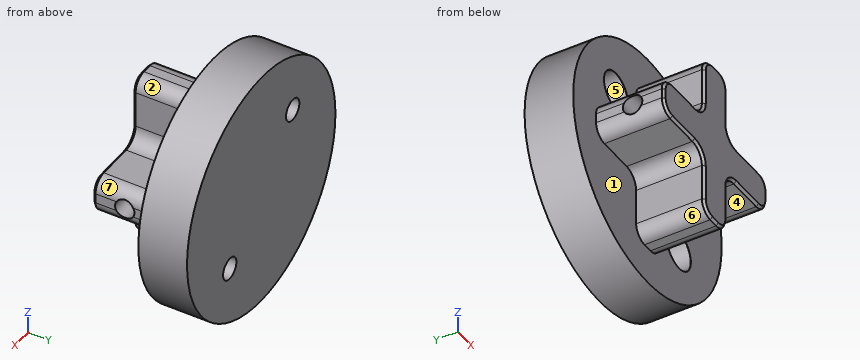
from build123d import *

# Parameters (mm, degrees)
SKETCH1_R                                    = 25
BOSS_EXTRUDE1_DEPTH                          = 25
BOSS_EXTRUDE2_DEPTH                          = 14
SKETCH3_R                                    = 2
CUT_EXTRUDE1_DEPTH                           = 56.129756031
CHAMFER1_SIZE                                = 0.5
CUT_EXTRUDE3_DEPTH                           = 15
CBORE_FOR_M4_HEX_SOCKET_HEAD_CAP_SCR_2_COUNT = 2
CBORE_FOR_M4_HEX_SOCKET_HEAD_CAP_SCR_2_PITCH = 30
CUT_EXTRUDE4_START                           = -15
CUT_EXTRUDE4_DEPTH                           = 15


with BuildPart() as part:
    # Sketch1 → Boss-Extrude1 (new body)
    with BuildSketch(Plane(origin=(0, 0, 0), x_dir=(1, 0, 0), z_dir=(0, 1, 0))):
        with Locations(Location((0, 0, 0), (0, 0, 270))):
            Circle(SKETCH1_R)
    extrude(amount=BOSS_EXTRUDE1_DEPTH)

    # Sketch2 → Boss-Extrude2 (add)
    with BuildSketch(Plane.XZ):
        with BuildLine():
            Line((-17.3, 1), (-17.3, -1))
            ThreePointArc((-17.3, -1), (-16.479898987, -2.979898987), (-14.5, -3.8))
            Line((-14.5, -3.8), (-7, -3.8))
            ThreePointArc((-7, -3.8), (-4.7372583, -4.7372583), (-3.8, -7))
            Line((-3.8, -7), (-3.8, -14.5))
            ThreePointArc((-3.8, -14.5), (-2.979898987, -16.479898987), (-1, -17.3))
            Line((-1, -17.3), (1, -17.3))
            ThreePointArc((1, -17.3), (2.979898987, -16.479898987), (3.8, -14.5))
            Line((3.8, -14.5), (3.8, -7))
            ThreePointArc((3.8, -7), (4.7372583, -4.7372583), (7, -3.8))
            Line((7, -3.8), (14.5, -3.8))
            ThreePointArc((14.5, -3.8), (16.479898987, -2.979898987), (17.3, -1))
            Line((17.3, -1), (17.3, 1))
            ThreePointArc((17.3, 1), (16.479898987, 2.979898987), (14.5, 3.8))
            Line((14.5, 3.8), (7, 3.8))
            ThreePointArc((7, 3.8), (4.7372583, 4.7372583), (3.8, 7))
            Line((3.8, 7), (3.8, 14.5))
            ThreePointArc((3.8, 14.5), (2.979898987, 16.479898987), (1, 17.3))
            Line((1, 17.3), (-1, 17.3))
            ThreePointArc((-1, 17.3), (-2.979898987, 16.479898987), (-3.8, 14.5))
            Line((-3.8, 14.5), (-3.8, 7))
            ThreePointArc((-3.8, 7), (-4.7372583, 4.7372583), (-7, 3.8))
            Line((-7, 3.8), (-14.5, 3.8))
            ThreePointArc((-14.5, 3.8), (-16.479898987, 2.979898987), (-17.3, 1))
        make_face()
    extrude(amount=BOSS_EXTRUDE2_DEPTH)

    # Sketch3 → Cut-Extrude1 (cut, through all)
    with BuildSketch(Plane.ZY.offset(17.3)):
        with Locations(Location((0, -7.5, 0), (0, 0, 60))):
            Circle(SKETCH3_R)
    extrude(amount=-CUT_EXTRUDE1_DEPTH, mode=Mode.SUBTRACT)

    # Chamfer1
    chamfer1_edges = [part.edges().sort_by_distance(p)[0] for p in [
        (-16.479898987, -14, -2.979898987),
        (-10.75, -14, -3.8),
        (-4.7372583, -14, -4.7372583),
        (-3.8, -14, -10.75),
        (-2.979898987, -14, -16.479898987),
        (0, -14, -17.3),
        (2.979898987, -14, -16.479898987),
        (3.8, -14, -10.75),
        (4.7372583, -14, -4.7372583),
        (10.75, -14, -3.8),
        (16.479898987, -14, -2.979898987),
        (17.3, -14, 0),
        (16.479898987, -14, 2.979898987),
        (10.75, -14, 3.8),
        (4.7372583, -14, 4.7372583),
        (3.8, -14, 10.75),
        (2.979898987, -14, 16.479898987),
        (0, -14, 17.3),
        (-2.979898987, -14, 16.479898987),
        (-3.8, -14, 10.75),
        (-4.7372583, -14, 4.7372583),
        (-10.75, -14, 3.8),
        (-16.479898987, -14, 2.979898987),
        (-17.3, -14, 0),
    ]]
    chamfer(chamfer1_edges, length=CHAMFER1_SIZE)

    # Sketch7 → Cut-Extrude3 (cut)
    with BuildSketch(Plane(origin=(0, 25, 0), x_dir=(1, 0, 0), z_dir=(0, 1, 0))):
        with BuildLine():
            Line((-25.358862505, -19.065612153), (19.065612153, 25.358862505))
            ThreePointArc((19.065612153, 25.358862505), (25.358862505, 25.358862505), (25.358862505, 19.065612153))
            Line((25.358862505, 19.065612153), (-19.065612153, -25.358862505))
            ThreePointArc((-19.065612153, -25.358862505), (-25.358862505, -25.358862505), (-25.358862505, -19.065612153))
        make_face()
    extrude(amount=-CUT_EXTRUDE3_DEPTH, mode=Mode.SUBTRACT)

    # Sketch6 → CBORE for M4 Hex Socket Head Cap Screw1 (revolve, cut)
    with BuildSketch(Plane(origin=(10.606601718, 0, -10.606601718), x_dir=(0, 0, -1), z_dir=(1, 0, 0))):
        Polygon((0, 0), (0, 14.351936393), (2.25, 13), (2.25, 4.4), (4, 4.4), (4, 0.025), (4.025, 0), align=None)
    cbore_for_m4_hex_socket_head_cap_screw1 = revolve(axis=Axis((10.606601718, -6.35, -10.606601718), (0, 1, 0)), mode=Mode.SUBTRACT)

    # CBORE for M4 Hex Socket Head Cap Scr 2: CBORE for M4 Hex Socket Head Cap Screw1 ×2
    with Locations(*[Vector(-0.707106781186549, 0, 0.7071067811865461) * (i * CBORE_FOR_M4_HEX_SOCKET_HEAD_CAP_SCR_2_PITCH) for i in range(1, CBORE_FOR_M4_HEX_SOCKET_HEAD_CAP_SCR_2_COUNT)]):
        add(cbore_for_m4_hex_socket_head_cap_screw1, mode=Mode.SUBTRACT)

    # Sketch8 → Cut-Extrude4 (cut)
    with BuildSketch(Plane(origin=(0, 25, 0), x_dir=(1, 0, 0), z_dir=(0, 1, 0)).offset(CUT_EXTRUDE4_START)):
        with BuildLine():
            Line((20.541990938, 14.248740586), (-14.248740586, -20.541990938))
            ThreePointArc((-14.248740586, -20.541990938), (17.67766953, -17.67766953), (20.541990938, 14.248740586))
        make_face()
        with BuildLine():
            Line((-20.541990938, -14.248740586), (14.248740586, 20.541990938))
            ThreePointArc((14.248740586, 20.541990938), (-17.67766953, 17.67766953), (-20.541990938, -14.248740586))
        make_face()
    extrude(amount=CUT_EXTRUDE4_DEPTH, mode=Mode.SUBTRACT)


solid = part.part
Geometry: final body of the model. Coordinates: model frame, mm. Face numbers are marked on the shaded views. A direction names the side the tool comes from. Give positions to 0.01 mm unless a question says otherwise; leave off trailing zeros. Write each loop counter-clockwise with the first axis right and the second up, starting at its lowest first coordinate (ties: lowest second). Pieces come first, ordered by that corner, then holes. Notation, with made-up numbers: M 24.25,64 L 70.25,64 A14 ccw 70.25,69 Z; hole C 45,7.5 d7. An arc over 180 degrees is marked long. Answer in a Markdown table with one row per item. Add a question column.
(1) Section A-A on x = 0. Return loops of the section in (y, z).
(2) Mould query, pull axis Z, two halves, no side actions, for the marked faces 5, 6 and 7. Classes: +Z half, -Z half, draft (parallel to the pull), parting line (faces both ways), or undercut.
(3) Section D-D on y = -7.5. Return loops of the section in (x, z), and give its area (3 significant figures).
(4) First-contact query: pin 1 (2 mm diameter, centred on x = -10, z = 8, fed in from -Y); pin 2 (8 mm diameter, centred on x = -11.5, y = -5.5, fed in from -Z); pin 3 (2 mm diameter, centred on y = -5, z = -14.5, fed in from -X); pin 4 (2.5 mm diameter, centred on y = -7.5, z = 0, fed in from -X). Flat tips, straight axial feed; report the tip coordinate or a pass-through.
(5) Section C-C on y = -11.5. Return loops of the section in (x, z).
(6) Section B-B on z = 0. Return loops of the section in (x, y).
(7) Reachability of the marked faces 1, 2, 3 and 4 from +Z, -Z, +X, -X, +Y, -Y: full face, straight path, thin tool, end or side. Return the list, or none.
(8) Ray query, line 1 (Y direction, x = 9, z = 0); line 2 (Y direction, x = -17.5, z = -2); line 3 (Z direction, x = -14, y = -1.75). Return the intervals inside material, ascending.
Result set:
| question | item | result |
|---|---|---|
| 1 | outline | M -14,-16.8 L -13.5,-17.3 L 0,-17.3 L 0,-25 L 10,-25 L 10,25 L 0,25 L 0,17.3 L -13.5,17.3 L -14,16.8 Z; hole C -7.5,0 d4 |
| 2 | face 5 | undercut |
| 2 | face 6 | -Z half |
| 2 | face 7 | +Z half |
| 3 | outline | M -17.12,-2 A2.8 ccw -14.5,-3.8 L -7,-3.8 A3.2 cw -3.8,-7 L -3.8,-14.5 A2.8 ccw -1,-17.3 L 1,-17.3 A2.8 ccw 3.8,-14.5 L 3.8,-7 A3.2 cw 7,-3.8 L 14.5,-3.8 A2.8 ccw 17.12,-2 Z; M -17.12,2 L 17.12,2 A2.8 ccw 14.5,3.8 L 7,3.8 A3.2 cw 3.8,7 L 3.8,14.5 A2.8 ccw 1,17.3 L -1,17.3 A2.8 ccw -3.8,14.5 L -3.8,7 A3.2 cw -7,3.8 L -14.5,3.8 A2.8 ccw Z |
| 3 | area | 325 mm^2 |
| 4 | pin 1 | stops at y = 4.4 |
| 4 | pin 2 | stops at z = -3.8 |
| 4 | pin 3 | stops at x = -3.8 |
| 4 | pin 4 | passes through |
| 5 | outline | M -17.3,-1 A2.8 ccw -14.5,-3.8 L -7,-3.8 A3.2 cw -3.8,-7 L -3.8,-14.5 A2.8 ccw -1,-17.3 L 1,-17.3 A2.8 ccw 3.8,-14.5 L 3.8,-7 A3.2 cw 7,-3.8 L 14.5,-3.8 A2.8 ccw 17.3,-1 L 17.3,1 A2.8 ccw 14.5,3.8 L 7,3.8 A3.2 cw 3.8,7 L 3.8,14.5 A2.8 ccw 1,17.3 L -1,17.3 A2.8 ccw -3.8,14.5 L -3.8,7 A3.2 cw -7,3.8 L -14.5,3.8 A2.8 ccw -17.3,1 Z |
| 6 | outline | M -25,0 L -17.3,0 L -17.3,-5.5 L 17.3,-5.5 L 17.3,0 L 25,0 L 25,10 L -25,10 Z; M -17.3,-13.5 L -16.8,-14 L 16.8,-14 L 17.3,-13.5 L 17.3,-9.5 L -17.3,-9.5 Z |
| 7 | face 1 | -Y |
| 7 | face 2 | +Z, +X, -Y |
| 7 | face 3 | -Z, -X, -Y |
| 7 | face 4 | -Z, +X, -Y |
| 8 | line 1 | y = -14 to -9.5, -5.5 to 10 |
| 8 | line 2 | y = 0 to 10 |
| 8 | line 3 | z = -3.8 to 3.8 |
